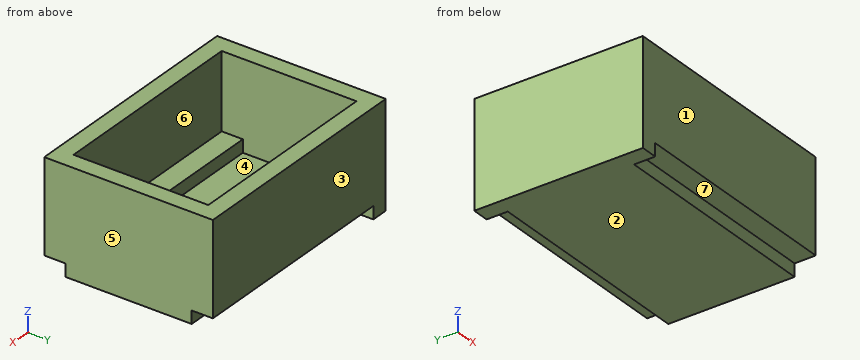
from build123d import *

# Parameters (mm, degrees)
SKETCH2_W           = 19.9273
SKETCH2_H           = 28
BOSS_EXTRUDE1_DEPTH = 12.4298
SKETCH3_W           = 2.5
SKETCH3_H           = 1.5
CUT_EXTRUDE1_DEPTH  = 26
SHELL1_START        = -12
SHELL1_DEPTH        = 24


# Read off the part's stored shape, not the designer's step: Shell1
with BuildPart() as part:
    # Sketch2 → Boss-Extrude1 (new body)
    with BuildSketch(Plane(origin=(0, 0, 0), x_dir=(0, 1, 0), z_dir=(0, 0, 1))):
        Rectangle(SKETCH2_W, SKETCH2_H)
    extrude(amount=BOSS_EXTRUDE1_DEPTH)

    # Sketch3 → Cut-Extrude1 (cut)
    with BuildSketch(Plane.YZ.offset(14)):
        with Locations((-8.71365, 0.75)):
            Rectangle(SKETCH3_W, SKETCH3_H)
        with Locations((8.71365, 0.75)):
            Rectangle(SKETCH3_W, SKETCH3_H)
    extrude(amount=-CUT_EXTRUDE1_DEPTH, mode=Mode.SUBTRACT)

    # Shell1 outline → Shell1 (cut)
    with BuildSketch(Plane.YZ.offset(SHELL1_START)):
        Polygon((7.96365, 3.5), (7.96365, 12.4298), (-7.96365, 12.4298), (-7.96365, 3.5), (-5.46365, 3.5), (-5.46365, 2), (5.46365, 2), (5.46365, 3.5), align=None)
    extrude(amount=SHELL1_DEPTH, mode=Mode.SUBTRACT)


solid = part.part
Part model, mm, in its own coordinate system. Face numbers are marked on the shaded views. A direction names the side the tool comes from. Coordinates: 2 decimals unless noted, no trailing zeros. Loops run counter-clockwise (first coordinate to the right, second up) from the corner with the lowest first, then second, coordinate; pieces in that order, holes last. Notation, with made-up numbers: (81.5, 24.5) -> (139.5, 24.5) arc R10 cw to (139.5, 38.5) -> close; hole circle Ø11 at (45, -39). An arc over 180 degrees is marked (long way). Use a Markdown table: item, result. Add a question column.
Item 1: Band-saw the part on D-D on z = 9. Write the cut outline in (x, y).
Item 2: Pull direction Y, two halves, no side cores. Call the marked faces 1, 2, 3 and 4: +Y half, -Y half, draft (parallel to the pull), parting line (faces both ways), or undercut.
Item 3: Band-saw the part on C-C on x = 5.75. Write the cut outline in (y, z), plus the area to 3 significant figures.
Item 4: Band-saw the part on B-B on y = -6.75. Write the cut outline in (x, z).
Item 5: Flat gauge pins, fed straight in: P1, Ø1.2, axis at x = -0.5, y = 8.5, coming from the -Z side; P2, Ø1.6, axis at y = 8.5, z = 0.5, coming from the +X side; P3, Ø0.8, axis at x = 4, z = 0.5, coming from the -Y side. Where does each tip first touch, or does it go through?
Item 6: Band-saw the part on A-A on z = 2.5. Write the cut outline in (x, y), plus the area to 3 significant figures.
Item 7: Probe probe 1 along Y at (x, z) = (-6.5, 4.75); probe 2 along X at (y, z) = (5, 6); probe 3 along Y at (x, z) = (9.75, 2.5). List the from-to ranges inside material, lowest first.
Item 8: Which spindle directions (+Z, -Z, +X, -X, +Y, -Y) get a long thin tool onto all of the face, cutting with end or side? Do the marked faces 5, 6 and 7. Say none if no direction does.
Geometry says:
| question | item | result |
|---|---|---|
| 1 | outline | (-14, -9.96) -> (14, -9.96) -> (14, 9.96) -> (-14, 9.96) -> close; hole (-12, -7.96) -> (12, -7.96) -> (12, 7.96) -> (-12, 7.96) -> close |
| 2 | face 1 | -Y half |
| 2 | face 2 | draft |
| 2 | face 3 | +Y half |
| 2 | face 4 | undercut |
| 3 | outline | (-9.96, 1.5) -> (-7.46, 1.5) -> (-7.46, 0) -> (7.46, 0) -> (7.46, 1.5) -> (9.96, 1.5) -> (9.96, 12.43) -> (7.96, 12.43) -> (7.96, 3.5) -> (5.46, 3.5) -> (5.46, 2) -> (-5.46, 2) -> (-5.46, 3.5) -> (-7.96, 3.5) -> (-7.96, 12.43) -> (-9.96, 12.43) -> close |
| 3 | area | 81.6 mm² |
| 4 | outline | (-14, 0) -> (14, 0) -> (14, 12.43) -> (12, 12.43) -> (12, 3.5) -> (-12, 3.5) -> (-12, 12.43) -> (-14, 12.43) -> close |
| 5 | P1 | z = 1.5 |
| 5 | P2 | x = -12 |
| 5 | P3 | y = -7.46 |
| 6 | outline | (-14, -9.96) -> (14, -9.96) -> (14, 9.96) -> (-14, 9.96) -> close; hole (-12, -5.46) -> (12, -5.46) -> (12, 5.46) -> (-12, 5.46) -> close |
| 6 | area | 296 mm² |
| 7 | probe 1 | -9.96 to -7.96, 7.96 to 9.96 |
| 7 | probe 2 | -14 to -12, 12 to 14 |
| 7 | probe 3 | -9.96 to -5.46, 5.46 to 9.96 |
| 8 | face 5 | +Z, -Z, +X, +Y, -Y |
| 8 | face 6 | +Z |
| 8 | face 7 | -Z, +X, -Y |
